```python
from build123d import *

# Parameters (mm, degrees)
SKETCH1_W               = 8
SKETCH1_H               = 8
BOSS_EXTRUDE1_DEPTH     = 3
CUT_EXTRUDE1_DEPTH      = 12.704699911
CUT_EXTRUDE1_DEPTH_BACK = 12.704699911
CUT_EXTRUDE2_DEPTH      = 11
SKETCH4_R               = 1.75
CUT_EXTRUDE3_DEPTH      = 0.4
SKETCH5_W               = 8
SKETCH5_H               = 1
BOSS_EXTRUDE2_DEPTH     = 2
FILLET1_R               = 4
CUT_EXTRUDE4_DEPTH      = 0.4


with BuildPart() as part:
    # Sketch1 → Boss-Extrude1 (new body)
    with BuildSketch(Plane(origin=(0, 0, 0), x_dir=(1, 0, 0), z_dir=(0, 1, 0))):
        with Locations((4, 4)):
            Rectangle(SKETCH1_W, SKETCH1_H)
    extrude(amount=BOSS_EXTRUDE1_DEPTH)

    # Sketch2 → Cut-Extrude1 (cut, two sides: drawn at the far end of the back side and taken through both)
    with BuildSketch(Plane.XY.offset(-CUT_EXTRUDE1_DEPTH_BACK)):
        Polygon((0, 0), (0.6, 3), (0, 3), align=None)
        Polygon((8, 0), (7.4, 3), (8, 3), align=None)
    extrude(amount=CUT_EXTRUDE1_DEPTH + CUT_EXTRUDE1_DEPTH_BACK, mode=Mode.SUBTRACT)

    # Sketch3 → Cut-Extrude2 (cut)
    with BuildSketch(Plane(origin=(0, 0, 0), x_dir=(0, 0, -1), z_dir=(1, 0, 0))):
        Polygon((0, 0), (0.6, 3), (0, 3), align=None)
        Polygon((8, 3), (7.4, 3), (8, 0), align=None)
    extrude(amount=CUT_EXTRUDE2_DEPTH, mode=Mode.SUBTRACT)

    # Sketch4 → Cut-Extrude3 (cut)
    with BuildSketch(Plane.XZ):
        with Locations(Location((4, -3.75, 0), (0, 0, 270))):
            Circle(SKETCH4_R)
    extrude(amount=-CUT_EXTRUDE3_DEPTH, mode=Mode.SUBTRACT)

    # Sketch5 → Boss-Extrude2 (add)
    with BuildSketch(Plane.XZ):
        with Locations((4, -7.5)):
            Rectangle(SKETCH5_W, SKETCH5_H)
    extrude(amount=BOSS_EXTRUDE2_DEPTH)

    # Fillet1
    # the kernel refuses this fillet: 4 mm, written as the material it takes off along each edge
    with BuildSketch(Plane(origin=(8, -2, -16.660254038), x_dir=(0, 1, 0), z_dir=(0, 0, 1)), Plane(origin=(0, -2, 1.660254038), x_dir=(0, 1, 0), z_dir=(0, 0, -1))) as fillet1_piece_1:
        with BuildLine():
            CenterArc((4, 3.464101615), FILLET1_R, 180, 60)
            Line((0, 3.464101615), (-0.08, 3.464101615))
            Line((-0.08, 3.464101615), (-0.08, 0))
            Line((-0.08, 0), (0, -0.08))
            ThreePointArc((0, -0.08), (1, -0.08), (1.96, -0.069282032))
            Line((1.96, -0.069282032), (2, 0))
        make_face()
    extrude(amount=18.320508076, mode=Mode.SUBTRACT)

    # Sketch6 → Cut-Extrude4 (cut)
    with BuildSketch(Plane(origin=(0, 3, 0), x_dir=(1, 0, 0), z_dir=(0, 1, 0))):
        Polygon((2.136477101, 1.987434605), (3.507470691, 4.106024349), (2.290323255, 5.987434605), (3.189361717, 5.987434605), (3.956989922, 4.800735887), (4.724618127, 5.987434605), (5.623656589, 5.987434605), (4.406509153, 4.106024349), (5.777502742, 1.987434605), (4.878464281, 1.987434605), (3.956989922, 3.41131281), (3.035515563, 1.987434605), align=None)
    extrude(amount=-CUT_EXTRUDE4_DEPTH, mode=Mode.SUBTRACT)


solid = part.part
```
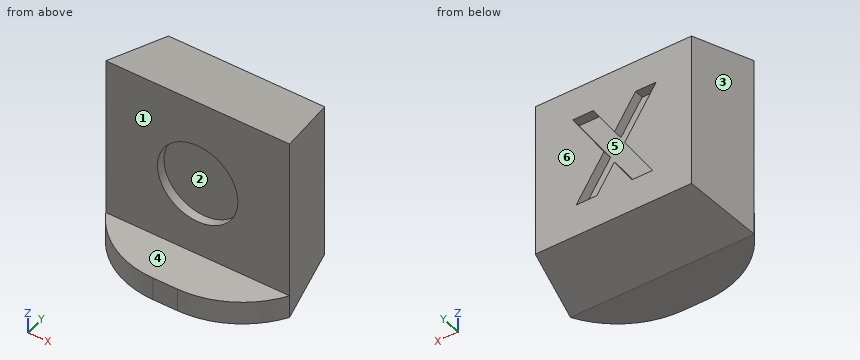
Geometry: final body of the model. Coordinates: model frame, mm. Face numbers are marked on the shaded views. A direction names the side the tool comes from. Coordinates: 2 decimals unless noted, no trailing zeros. Order: outer loops, then holes, each group sorted by start corner. A loop starts at its lowest first (then second) coordinate and runs counter-clockwise, first axis right, second up. Notation, with made-up numbers: M 13,-28.5 L 33,-28.5 A20 ccw 33,-23.5 Z; hole C 19.5,-28.5 d9. An arc over 180 degrees is marked long. Answer in a Markdown table with one row per item. Add a question column.
Q1. Section query C-C on z = -6.25. Return the cut outline in (x, y).
Q2. Reachability of the marked faces 4, 5 and 6 from +Z, -Z, +X, -X, +Y, -Y: full face, straight path, thin tool, end or side. Return the list, or none.
Q3. Section query A-A on y = 0.3. Return the cut outline in (x, z), and give its area (3 significant figures).
Q4. Line query: L1, parallel to Z at x = 5, y = -0.95; L2, parallel to Y at x = 5.75, z = -1; L3, parallel to Y at x = 5, z = -3.5. Output: solid intervals per line, ascending.
Q5. Contact query for flat-ended pins moving along their axis: P1, Ø2, axis at y = 2, z = -6.5, coming from the +X side; P2, Ø1, axis at x = 1, y = 2, coming from the -Z side; P3, Ø2, axis at y = -1.5, z = -5.5, coming from the -X side; P4, Ø1.6, axis at x = 5.5, y = -1, coming from the +Z side. Output: stop coordinate, or through.
Q6. Section query D-D on y = 1.7. Return the cut outline in (x, z), and give its area (3 significant figures).
Q7. Mould query, pull axis X, two halves, no side actions, for the marked faces 1, 2 and 3. Classes: released by +X, released by -X, zero draft, split by the parting line, or undercut.
Q8. Section query B-B on x = 6.5. Return the cut outline in (y, z).
Completed:
| question | item | result |
|---|---|---|
| 1 | outline | M 0,0 L 8,0 L 7.4,3 L 0.6,3 Z |
| 2 | face 4 | +Z, +X, -X, -Y |
| 2 | face 5 | +Y |
| 2 | face 6 | +Z, -Z, +X, -X, +Y |
| 3 | outline | M 0.06,-7.94 L 7.94,-7.94 L 7.94,-0.06 L 0.06,-0.06 Z; hole C 4,-3.75 d3.5 |
| 3 | area | 52.5 mm2 |
| 4 | L1 | z = -8 to -7 |
| 4 | L2 | y = 0 to 3 |
| 4 | L3 | y = 0.4 to 3 |
| 5 | P1 | stops at x = 7.8 |
| 5 | P2 | stops at z = -7.7 |
| 5 | P3 | passes through |
| 5 | P4 | stops at z = -7 |
| 6 | outline | M 0.34,-7.66 L 7.66,-7.66 L 7.66,-0.34 L 0.34,-0.34 Z |
| 6 | area | 53.6 mm2 |
| 7 | face 1 | zero draft |
| 7 | face 2 | undercut |
| 7 | face 3 | released by -X |
| 8 | outline | M -1.48,-8 L 0,-8 L 3,-7.4 L 3,-0.6 L 0,0 L 0,-7 L -1.48,-7 Z |
